```python
from build123d import *

# Parameters (mm, degrees)
SKETCH1_R           = 50.5
BOSS_EXTRUDE1_DEPTH = 5
SKETCH3_R           = 1.75
BOSS_EXTRUDE2_DEPTH = 10
SKETCH4_R           = 1.7
SKETCH4_R_2         = 3.2639
CUT_EXTRUDE2_DEPTH  = 73.114492302
SKETCH5_R           = 4.826
CUT_EXTRUDE3_DEPTH  = 73.114492302
SKETCH6_R           = 1
CUT_EXTRUDE4_DEPTH  = 10
FILLET1_R           = 3
SKETCH7_R           = 4.5
CUT_EXTRUDE5_DEPTH  = 73.97602346


with BuildPart() as part:
    # Sketch1 → Boss-Extrude1 (new body)
    with BuildSketch(Plane(origin=(0, 0, 0), x_dir=(1, 0, 0), z_dir=(0, 1, 0))):
        with Locations(Location((0, 0, 0), (0, 0, 270))):
            Circle(SKETCH1_R)
    extrude(amount=BOSS_EXTRUDE1_DEPTH)

    # Sketch3 → Boss-Extrude2 (add)
    with BuildSketch(Plane(origin=(0, 5, 0), x_dir=(1, 0, 0), z_dir=(0, 1, 0))):
        Polygon((0, -14.849242405), (14.849242405, 0), (0, 14.849242405), (-14.849242405, 0), align=None)
        with Locations(Location((10, 0, 0), (0, 0, 270))):
            Circle(SKETCH3_R, mode=Mode.SUBTRACT)
        with Locations(Location((0, -10, 0), (0, 0, 270))):
            Circle(SKETCH3_R, mode=Mode.SUBTRACT)
        with Locations(Location((-10, 0, 0), (0, 0, 270))):
            Circle(SKETCH3_R, mode=Mode.SUBTRACT)
        with Locations(Location((0, 10, 0), (0, 0, 270))):
            Circle(SKETCH3_R, mode=Mode.SUBTRACT)
    extrude(amount=BOSS_EXTRUDE2_DEPTH)

    # Sketch4 → Cut-Extrude2 (cut, through all)
    with BuildSketch(Plane(origin=(0, 5, 0), x_dir=(1, 0, 0), z_dir=(0, 1, 0))):
        with Locations(Location((21.213203436, 21.213203436, 0), (0, 0, 270))):
            Circle(SKETCH4_R)
        with Locations(Location((-21.213203436, -21.213203436, 0), (0, 0, 90))):
            Circle(SKETCH4_R)
        with Locations(Location((-24.748737342, 24.748737342, 0), (0, 0, 270))):
            Circle(SKETCH4_R_2)
        with Locations(Location((24.748737342, -24.748737342, 0), (0, 0, 90))):
            Circle(SKETCH4_R_2)
    extrude(amount=-CUT_EXTRUDE2_DEPTH, mode=Mode.SUBTRACT)

    # Sketch5 → Cut-Extrude3 (cut, through all)
    with BuildSketch(Plane(origin=(0, 5, 0), x_dir=(1, 0, 0), z_dir=(0, 1, 0))):
        with Locations(Location((34, 0, 0), (0, 0, 270))):
            Circle(SKETCH5_R)
        with Locations(Location((0, 34, 0), (0, 0, 270))):
            Circle(SKETCH5_R)
        with Locations(Location((-34, 0, 0), (0, 0, 270))):
            Circle(SKETCH5_R)
        with Locations(Location((0, -34, 0), (0, 0, 270))):
            Circle(SKETCH5_R)
    extrude(amount=-CUT_EXTRUDE3_DEPTH, mode=Mode.SUBTRACT)

    # Sketch6 → Cut-Extrude4 (cut)
    with BuildSketch(Plane(origin=(0, 5, 0), x_dir=(1, 0, 0), z_dir=(0, 1, 0))):
        with Locations(Location((0, 21, 0), (0, 0, 270))):
            Circle(SKETCH6_R)
        with Locations(Location((-21, 0, 0), (0, 0, 270))):
            Circle(SKETCH6_R)
        with Locations(Location((21, 0, 0), (0, 0, 270))):
            Circle(SKETCH6_R)
        with Locations(Location((0, -21, 0), (0, 0, 270))):
            Circle(SKETCH6_R)
    extrude(amount=-CUT_EXTRUDE4_DEPTH, mode=Mode.SUBTRACT)

    # Fillet1
    fillet1_edges = [part.edges().sort_by_distance(p)[0] for p in [
        (-14.849242405, 10, 0),
        (0, 10, 14.849242405),
        (14.849242405, 10, 0),
        (0, 10, -14.849242405),
    ]]
    fillet(fillet1_edges, radius=FILLET1_R)

    # Sketch7 → Cut-Extrude5 (cut, through all)
    with BuildSketch(Plane(origin=(0, 0, 0), x_dir=(1, 0, 0), z_dir=(0, 1, 0))):
        with Locations(Location((-22, 38.105117767, 0), (0, 0, 270))):
            Circle(SKETCH7_R)
    extrude(amount=CUT_EXTRUDE5_DEPTH, mode=Mode.SUBTRACT)


solid = part.part
```
Read the model definition and answer for the solid it produces. Units are mm, in the model's axes. A direction names the side the tool comes from. Give positions to 0.01 mm unless a question says otherwise; leave off trailing zeros. Write each loop counter-clockwise with the first axis right and the second up, starting at its lowest first coordinate (ties: lowest second). Pieces come first, ordered by that corner, then holes. Notation, with made-up numbers: (89, 55) - (118, 55) arc R14 cw to (118, 67) - close; hole circle Ø1 at (64, 77.5). An arc over 180 degrees is marked (long way). Write item = value, one per line. Start each with the question number.
Item 1: Find section D-D (z = -10). Give the vertices of the cut face in (x, y).
Item 2: The mould has two halves that part along Z. Classify faces 6 (the flat face through (7.35, 9.93, 7.5)), 7 (the cylindrical face through (0.033, 10.07, -13.606)), 8 (the flat face through (0, 5, -10)): +Z half, -Z half, draft (parallel to the pull), parting line (faces both ways), or undercut.
Item 3: Find section A-A (x = -34). Give the vertices of the cut face in (y, z).
Item 4: Find the intervals of material crossed by probe 1 along X at (y, z) = (1.7, 0); probe 2 along X at (y, z) = (8.5, -10); probe 3 along X at (y, z) = (8.5, 0), in increasing order. Write a range as [from, to].
Item 5: Each of these flat-tipped pins is pushed along its axis until it touches: P1, Ø1.8, axis at x = 0.5, z = 10, coming from the +Y side; P2, Ø5, axis at y = 3, z = 23.5, coming from the -X side. Where does it stop, or does it pass through?
Item 6: Find section B-B (y = 13.25). Give the vertices of the cut face in (x, z).
Item 7: Find section C-C (y = 2.75). State how many separate pieces and enclosed holes the cut face has, then the cut area to 3 significant figures.
Item 8: A tool of negligible diameter and unlimited length cuts with its end or side. For faces 1 (the flat face through (-7.35, 9.93, -7.5)), 2 (the cylindrical face through (0.033, 10.07, 13.606)), 3 (the flat face through (10, 5, 0)), 4 (the cylindrical face through (-13.606, 10.07, 0.033)), 5 (the flat face through (7.5, 9.93, -7.35)), from which of +Z, -Z, +X, -X, +Y, -Y can it reach the whole face along a straight path? Write none if from no direction.
Response:
q1.outline = (-49.5, 0) - (49.5, 0) - (49.5, 5) - (4.85, 5) - (4.85, 15) - (1.75, 15) - (1.75, 5) - (-1.75, 5) - (-1.75, 15) - (-4.85, 15) - (-4.85, 5) - (-49.5, 5) - close
q2.face_6 = +Z half
q2.face_7 = -Z half
q2.face_8 = undercut
q3.outline = (0, -37.34) - (5, -37.34) - (5, -4.83) - (0, -4.83) - close; (0, 4.83) - (5, 4.83) - (5, 37.34) - (0, 37.34) - close
q4.probe_1 = [-50.5, -38.83], [-29.17, -22], [-20, 20], [22, 29.17], [38.83, 50.5]
q4.probe_2 = [-4.85, -1.75], [1.75, 4.85]
q4.probe_3 = [-13.61, -11.75], [-8.25, 8.25], [11.75, 13.61]
q5.P1 = 5
q5.P2 = -45.93
q6.outline = (-12.73, -2.12) - (-2.12, -12.73) arc R3 ccw to (2.12, -12.73) - (12.73, -2.12) arc R3 ccw to (12.73, 2.12) - (2.12, 12.73) arc R3 ccw to (-2.12, 12.73) - (-12.73, 2.12) arc R3 ccw to start; hole circle Ø3.5 at (-10, 0); hole circle Ø3.5 at (0, -10); hole circle Ø3.5 at (0, 10); hole circle Ø3.5 at (10, 0)
q7.separate_pieces = 1
q7.enclosed_holes = 13
q7.area = 7,560 mm²
q8.face_1 = -Z, -X, +Y
q8.face_2 = +Z, +Y
q8.face_3 = +Y
q8.face_4 = -X, +Y
q8.face_5 = -Z, +X, +Y
